Work out the finished part from the listing and answer in its coordinate system (mm). A direction names the side the tool comes from. Round coordinates to 2 decimals unless told otherwise and drop trailing zeros. Write each loop counter-clockwise with the first axis right and the second up, starting at its lowest first coordinate (ties: lowest second). Pieces come first, ordered by that corner, then holes. Notation, with made-up numbers: M 67,-33.75 L 73,-33.75 A30 ccw 73,-10.75 Z; hole C 41,-24.75 d3. An arc over 180 degrees is marked long. Answer in a Markdown table with one row per item.
```python
from build123d import *

# Parameters (mm, degrees)
SKETCH1_W                      = 22
SKETCH1_H                      = 28
BOSS_EXTRUDE1_DEPTH            = 1.66
SKETCH2_W                      = 5.16
SKETCH2_H                      = 4.3
BOSS_EXTRUDE2_DEPTH            = 1
F_2_6_2_6_DIAMETER_HOLE1_D     = 2.6
F_2_6_2_6_DIAMETER_HOLE1_DEPTH = 2.66
SKETCH6_R                      = 0.5
CUT_EXTRUDE1_DEPTH             = 18.881711327


with BuildPart() as part:
    # Sketch1 → Boss-Extrude1 (new body)
    with BuildSketch(Plane(origin=(0, 0.83, 0), x_dir=(1, 0, 0), z_dir=(0, 1, 0))):
        Rectangle(SKETCH1_W, SKETCH1_H)
    extrude(amount=-BOSS_EXTRUDE1_DEPTH)

    # Sketch2 → Boss-Extrude2 (add)
    with BuildSketch(Plane(origin=(0, 0.83, 0), x_dir=(-1, 0, 0), z_dir=(0, 1, 0))):
        with Locations((0, 6.5)):
            Rectangle(SKETCH2_W, SKETCH2_H)
    extrude(amount=BOSS_EXTRUDE2_DEPTH)

    # 2.6 _2.6_ Diameter Hole1
    with Locations(Plane(origin=(0, -0.83, 0), x_dir=(-1, 0, 0), z_dir=(0, -1, 0))):
        with Locations((9, -1), (-9, -1), (9, -12), (-9, -12)):
            Hole(F_2_6_2_6_DIAMETER_HOLE1_D / 2, depth=F_2_6_2_6_DIAMETER_HOLE1_DEPTH)

    # Sketch6 → Cut-Extrude1 (cut, through all)
    with BuildSketch(Plane(origin=(0, 0.83, 0), x_dir=(1, 0, 0), z_dir=(0, 1, 0))):
        with Locations(Location((-8.89, 10.508626005, 0), (0, 0, 270))):
            Circle(SKETCH6_R)
        with Locations(Location((-8.89, 7.968626005, 0), (0, 0, 270))):
            Circle(SKETCH6_R)
        with Locations(Location((-6.35, 10.508626005, 0), (0, 0, 270))):
            Circle(SKETCH6_R)
        with Locations(Location((-6.35, 7.968626005, 0), (0, 0, 270))):
            Circle(SKETCH6_R)
        with Locations(Location((-3.81, 10.508626005, 0), (0, 0, 270))):
            Circle(SKETCH6_R)
        with Locations(Location((-3.81, 7.968626005, 0), (0, 0, 270))):
            Circle(SKETCH6_R)
        with Locations(Location((-1.27, 10.508626005, 0), (0, 0, 270))):
            Circle(SKETCH6_R)
        with Locations(Location((-1.27, 7.968626005, 0), (0, 0, 270))):
            Circle(SKETCH6_R)
        with Locations(Location((1.27, 10.508626005, 0), (0, 0, 270))):
            Circle(SKETCH6_R)
        with Locations(Location((1.27, 7.968626005, 0), (0, 0, 270))):
            Circle(SKETCH6_R)
        with Locations(Location((3.81, 10.508626005, 0), (0, 0, 270))):
            Circle(SKETCH6_R)
        with Locations(Location((3.81, 7.968626005, 0), (0, 0, 270))):
            Circle(SKETCH6_R)
        with Locations(Location((6.35, 10.508626005, 0), (0, 0, 270))):
            Circle(SKETCH6_R)
        with Locations(Location((6.35, 7.968626005, 0), (0, 0, 270))):
            Circle(SKETCH6_R)
        with Locations(Location((8.89, 10.508626005, 0), (0, 0, 270))):
            Circle(SKETCH6_R)
        with Locations(Location((8.89, 7.968626005, 0), (0, 0, 270))):
            Circle(SKETCH6_R)
        with Locations(Location((-1.288362942, 3.232735908, 0), (0, 0, 270))):
            Circle(SKETCH6_R)
        with Locations(Location((1.251637058, 3.232735908, 0), (0, 0, 270))):
            Circle(SKETCH6_R)
        with Locations(Location((3.791637058, 3.232735908, 0), (0, 0, 270))):
            Circle(SKETCH6_R)
    extrude(amount=-CUT_EXTRUDE1_DEPTH, mode=Mode.SUBTRACT)


solid = part.part
```
1. Consider line 1 along Z through (x, y) = (4, -0.55); line 2 along Y through (x, z) = (8.5, -5.25); line 3 along X through (y, z) = (0.1, 2). Determine where each line is inside the solid, lowest interval first. Write a range as from..to.
Calculated:
| item | result |
|---|---|
| line 1 | z = -14..-10.97, -10.05..-8.43, -7.51..-3.69, -2.78..14 |
| line 2 | y = -0.83..0.83 |
| line 3 | x = -11..-9.83, -8.17..8.17, 9.83..11 |
2. The part is cut by section B-B (x = -3.81). Determine the outline of the cut face in (y, z).
Calculated:
| item | result |
|---|---|
| outline | M -0.83,-14 L 0.83,-14 L 0.83,-11.01 L -0.83,-11.01 Z; M -0.83,-10.01 L 0.83,-10.01 L 0.83,-8.47 L -0.83,-8.47 Z; M -0.83,-7.47 L 0.83,-7.47 L 0.83,14 L -0.83,14 Z |
3. A tool of negligible diameter and unlimited length cuts with its end or side. For faces 1 (the flat face through (0, 0, 14)), 2 (the cylindrical face through (3.814, 0.012, -3.732)), 3 (the flat face through (-2.58, 1, 6)), 4 (the flat face through (0, 1, 4.35)), 5 (the flat face through (2.58, 1, 6)), from which of +Z, -Z, +X, -X, +Y, -Y can it reach the whole face along a straight path? Write none if from no direction.
Calculated:
| item | result |
|---|---|
| face 1 | +Z, +X, -X, +Y, -Y |
| face 2 | +Y, -Y |
| face 3 | +Z, -Z, -X, +Y |
| face 4 | -Z, +X, -X, +Y |
| face 5 | +Z, -Z, +X, +Y |
4. Given pin 1 (6.5 mm diameter, centred on x = -1.5, z = -6, fed in from +Y); pin 2 (0.8 mm diameter, centred on x = 0.5, y = 1.5, fed in from +Z), each flat-ended and moving along its own axis, determine where each tip first touches the part or whether it passes through.
Calculated:
| item | result |
|---|---|
| pin 1 | stops at y = 0.83 |
| pin 2 | stops at z = 8.65 |
5. The part is cut by section C-C (y = -0.1). Count the separate pieces of the cut face and the enclosed holes in it, plus the area to 3 significant figures.
Calculated:
| item | result |
|---|---|
| separate pieces | 1 |
| enclosed holes | 23 |
| area | 580 mm² |
6. The part is cut by section A-A (z = 1). Determine the outline of the cut face in (x, y), plus the area to 3 significant figures.
Calculated:
| item | result |
|---|---|
| outline | M -11,-0.83 L -10.3,-0.83 L -10.3,0.83 L -11,0.83 Z; M -7.7,-0.83 L 7.7,-0.83 L 7.7,0.83 L -7.7,0.83 Z; M 10.3,-0.83 L 11,-0.83 L 11,0.83 L 10.3,0.83 Z |
| area | 27.9 mm² |
7. Determine the mould class of faces 6 (the flat face through (11, 0, 0)), 7 (the cylindrical face through (-1.25, 0.01, -8.47)), 8 (the flat face through (0, 0, -14)) for opening direction X: released by +X, released by -X, zero draft, split by the parting line, or undercut.
Calculated:
| item | result |
|---|---|
| face 6 | released by +X |
| face 7 | undercut |
| face 8 | zero draft |
8. The part is cut by section D-D (y = 1.4). Determine the outline of the cut face in (x, z).
Calculated:
| item | result |
|---|---|
| outline | M -2.58,4.35 L 2.58,4.35 L 2.58,8.65 L -2.58,8.65 Z |
